The listing builds one solid part. Answer for the finished solid, in the listing's coordinates (mm). Face numbers are marked on the shaded views. A direction names the side the tool comes from. Give positions to 0.01 mm unless a question says otherwise; leave off trailing zeros. Write each loop counter-clockwise with the first axis right and the second up, starting at its lowest first coordinate (ties: lowest second). Pieces come first, ordered by that corner, then holes. Notation, with made-up numbers: (26, -38.5) - (83, -38.5) arc R29 cw to (83, -10.5) - close; hole circle Ø9 at (26, -8.75). An arc over 180 degrees is marked (long way). One line per question, with ' | ' between items. Start each with the question number.
1. A cutting plane is placed at B-B (y = 11.5). Determine the outline of the cut face in (x, z), then the cut area to 3 significant figures.
2. A cutting plane is placed at C-C (z = 5). Determine the outline of the cut face in (x, y), then the cut area to 3 significant figures.
3. A cutting plane is placed at A-A (z = 10.8). Determine the outline of the cut face in (x, y).
4. Find the intervals of material crossed by L1, parallel to X at y = 12, z = 17; L2, parallel to Z at x = -17.5, y = -7.5; L3, parallel to Y at x = -2.2, z = -19.2, in increasing order. Write a range as from..to.
5. Given P1, Ø3.5, axis at x = 21.5, y = 2, coming from the -Z side; P2, Ø7, axis at y = 10.69, z = -19.2, coming from the -X side; P3, Ø11, axis at y = 7.5, z = -20, coming from the +X side, each flat-ended and moving along its own axis, determine where each tip first touches the part or whether it passes through.
6. For the marked faces 1, 2, 3 and 4, determine the directions among +Z, -Z, +X, -X, +Y, -Y from which every point of the face is accessible in a straight line to the end or side of a thin tool.
7. A cutting plane is placed at D-D (x = 11). Determine the outline of the cut face in (y, z), then the cut area to 3 significant figures.
8. The mould has two halves that part along X. Classify the marked faces 5, 6, 7 and 8: +X half, -X half, draft (parallel to the pull), parting line (faces both ways), or undercut.
```python
from build123d import *

# Parameters (mm, degrees)
SKETCH1_R                    = 4
SKETCH1_R_2                  = 2.249999999999999
BOSS_EXTRUDE1_DEPTH          = 24
SKETCH2_R                    = 2.2499999999999956
SKETCH2_R_2                  = 4
BOSS_EXTRUDE2_DEPTH          = 24
CUT_EXTRUDE1_DEPTH           = 14
CUT_EXTRUDE2_START           = -14
CUT_EXTRUDE2_DEPTH           = 14
BOSS_EXTRUDE3_DEPTH          = 2
CUT_EXTRUDE_THIN1_DEPTH      = 70.97528134991671
CUT_EXTRUDE_THIN1_DEPTH_BACK = 53.00000000000001
SKETCH6_W                    = 2
SKETCH6_H                    = 35.40537681916631
SKETCH7_R                    = 2.249999999999999
CUT_EXTRUDE3_DEPTH           = 55.524673314014464
CUT_EXTRUDE4_DEPTH           = 41.99999999999999
CHAMFER2_SIZE                = 1
SKETCH9_R                    = 45.63024731549585
CUT_EXTRUDE5_DEPTH           = 2
SKETCH10_R                   = 89.28313808685371
CUT_EXTRUDE6_DEPTH           = 57.00000000000001
BOSS_EXTRUDE5_START          = 3
SKETCH11_R                   = 3.9999999999999925
BOSS_EXTRUDE5_DEPTH          = 3
BOSS_EXTRUDE6_DEPTH          = 3
BOSS_EXTRUDE7_DEPTH          = 3
CUT_EXTRUDE7_DEPTH           = 56.55663776723714
CUT_EXTRUDE7_DEPTH_BACK      = 56.55663776723714
CUT_EXTRUDE8_START           = -18.000000000000004
CUT_EXTRUDE8_DEPTH           = 18.000000000000004
CHAMFER4_SIZE                = 5


with BuildPart() as part:
    # Sketch1 → Boss-Extrude1 (new body)
    with BuildSketch(Plane.XY):
        with BuildLine():
            Line((0, 15.5), (-30, 15.5))
            Line((-30, 15.5), (-45.50000000000001, 15.499999999999995))
            Line((-45.50000000000001, 15.499999999999995), (-45.5, 1.9e-15))
            ThreePointArc((-45.5, 1.9e-15), (-40.96015510839149, -10.960155108391486), (-30, -15.499999999999996))
            Line((-30, -15.499999999999996), (0, -15.5))
            ThreePointArc((0, -15.5), (10.960155108391488, -10.960155108391486), (15.5, 0))
            Line((15.5, 0), (15.5, 15.5))
            Line((15.5, 15.5), (0, 15.5))
        make_face()
        Circle(SKETCH1_R, mode=Mode.SUBTRACT)
        with Locations((-30, 0)):
            Circle(SKETCH1_R_2, mode=Mode.SUBTRACT)
    extrude(amount=BOSS_EXTRUDE1_DEPTH)

    # Sketch4 → Cut-Extrude2 (cut)
    with BuildSketch(Plane.XY.offset(24).offset(CUT_EXTRUDE2_START)):
        with BuildLine():
            Line((-1.32e-15, 15.499999999999998), (-45.50000000000001, 15.499999999999995))
            Line((-45.50000000000001, 15.499999999999995), (-45.5, 1.9e-15))
            ThreePointArc((-45.5, 1.9e-15), (-40.96015510839149, -10.960155108391486), (-30.000000000000004, -15.5))
            Line((-30.000000000000004, -15.5), (0, -15.5))
            ThreePointArc((0, -15.5), (-15.499999999999998, 1.9e-15), (-1.32e-15, 15.499999999999998))
        make_face()
    extrude(amount=CUT_EXTRUDE2_DEPTH, mode=Mode.SUBTRACT)



with BuildPart() as body_2:
    # Sketch2 → Boss-Extrude2 (new body)
    with BuildSketch(Plane(origin=(0, 0, -2.2), x_dir=(-1, 0, 0), z_dir=(0, 0, -1))):
        with BuildLine():
            Line((-2.85e-15, -15.5), (30.000000000000004, -15.499999999999998))
            ThreePointArc((30.000000000000004, -15.499999999999998), (40.96015510839149, -10.960155108391485), (45.5, 0))
            Line((45.5, 0), (45.50000000000001, 15.499999999999995))
            Line((45.50000000000001, 15.499999999999995), (-15.5, 15.5))
            Line((-15.5, 15.5), (-15.5, 1.73e-15))
            ThreePointArc((-15.5, 1.73e-15), (-10.96015510839149, -10.960155108391486), (-2.85e-15, -15.5))
        make_face()
        with Locations((30, 0)):
            Circle(SKETCH2_R, mode=Mode.SUBTRACT)
        Circle(SKETCH2_R_2, mode=Mode.SUBTRACT)
    extrude(amount=BOSS_EXTRUDE2_DEPTH)

    # Sketch3 → Cut-Extrude1 (cut)
    with BuildSketch(Plane(origin=(0, 0, -26.200000000000003), x_dir=(-1, 0, 0), z_dir=(0, 0, -1))):
        with BuildLine():
            Line((-2.85e-15, -15.5), (30.000000000000004, -15.499999999999998))
            ThreePointArc((30.000000000000004, -15.499999999999998), (40.96015510839149, -10.960155108391485), (45.5, 0))
            Line((45.5, 0), (45.50000000000001, 15.499999999999995))
            Line((45.50000000000001, 15.499999999999995), (1.32e-15, 15.499999999999998))
            ThreePointArc((1.32e-15, 15.499999999999998), (15.5, -3.44e-15), (-2.85e-15, -15.5))
        make_face()
    extrude(amount=-CUT_EXTRUDE1_DEPTH, mode=Mode.SUBTRACT)


with BuildPart() as part_1:
    add(part.part)

    add(body_2.part)  # Boss-Extrude3 merges body 2
    # Sketch5 → Boss-Extrude3 (add)
    with BuildSketch(Plane(origin=(-1.32e-15, 15.499999999999998, 0), x_dir=(1, 1.1e-16, 0), z_dir=(-1.1e-16, 1, 0))):
        Polygon((-45.50000000000001, 12.200000000000001), (1.77e-15, 12.200000000000001), (0, 26.200000000000003), (15.500000000000002, 26.200000000000003), (15.500000000000002, -24), (0, -24), (1.77e-15, -10), (-45.50000000000001, -10), (-45.50000000000001, 0), (-38.50000000000001, 0), (-38.50000000000001, 2.200000000000001), (-45.50000000000001, 2.2), align=None)
    extrude(amount=BOSS_EXTRUDE3_DEPTH)

    # Chamfer1
    # the kernel refuses this chamfer: 10 mm, written as the material it adds along each edge
    with BuildSketch(Plane(origin=(-3.72e-15, 15.5, 10), x_dir=(0.026587242345483465, 0.9996464967899715, 0), z_dir=(0, 0, 1))) as chamfer1_piece_1_section:
        with BuildLine():
            Line((8.29406545002713, 1e-17), (-1.7422154358514688, 6.254838102034438))
            Line((-1.7422154358514688, 6.254838102034438), (-1.9240447967842007, 6.17154294309471))
            ThreePointArc((-1.9240447967842007, 6.17154294309471), (-0.6239231337177482, 3.187248798266774), (-0.19992929935799358, -0.00531744846909673))
            Line((-0.19992929935799358, -0.00531744846909673), (0.00531744846909669, -0.1999292993579943))
            ThreePointArc((0.00531744846909669, -0.1999292993579943), (4.149418712953845, -0.08971011189834381), (8.299382898496228, -0.19992929935799428))
            Line((8.299382898496228, -0.19992929935799428), (8.29406545002713, 1e-17))
        make_face()
    chamfer1_piece_1 = extrude(amount=14, mode=Mode.PRIVATE)
    chamfer1_piece_1 = split(chamfer1_piece_1, bisect_by=Plane(origin=(-2.6872969980278754, 17.5, 17.000000000000004), z_dir=(1.1e-16, -1, 0)), keep=Keep.TOP, mode=Mode.PRIVATE)
    add(chamfer1_piece_1)
    with BuildSketch(Plane(origin=(-1.32e-15, 15.5, -26.200000000000003), x_dir=(-0.9701220678115945, -0.24261733974503139, 0), z_dir=(0, 0, 1))) as chamfer1_piece_2_section:
        with BuildLine():
            Line((6.4929434240243395, 9e-17), (-2.2255005025199233, -7.9899104627409505))
            Line((-2.2255005025199233, -7.9899104627409505), (-2.419524916082242, -7.941386994791944))
            ThreePointArc((-2.419524916082242, -7.941386994791944), (-1.1998107866971348, -3.973182305874418), (-0.19402441356231892, 0.04852346794900628))
            Line((-0.19402441356231892, 0.04852346794900628), (0.0485234679490061, 0.1940244135623182))
            ThreePointArc((0.0485234679490061, 0.1940244135623182), (3.237781752513792, -0.25417376326036684), (6.461492077353489, 0.19751155103585727))
            Line((6.461492077353489, 0.19751155103585727), (6.4929434240243395, 9e-17))
        make_face()
    chamfer1_piece_2 = extrude(amount=14, mode=Mode.PRIVATE)
    chamfer1_piece_2 = split(chamfer1_piece_2, bisect_by=Plane(origin=(-2.687296998027888, 17.5, -19.200000000000006), z_dir=(1.1e-16, -1, 0)), keep=Keep.TOP, mode=Mode.PRIVATE)
    add(chamfer1_piece_2)

    # Sketch6 → Cut-Extrude-Thin1 (cut, two sides: drawn at the far end of the back side and taken through both)
    with BuildSketch(Plane(origin=(0, 0, -26.200000000000003), x_dir=(-1, 0, 0), z_dir=(0, 0, -1)).offset(-CUT_EXTRUDE_THIN1_DEPTH_BACK)):
        with Locations((0, 17.702688409583153)):
            Rectangle(SKETCH6_W, SKETCH6_H)
    extrude(amount=CUT_EXTRUDE_THIN1_DEPTH + CUT_EXTRUDE_THIN1_DEPTH_BACK, mode=Mode.SUBTRACT)

    # Sketch7 → Cut-Extrude3 (cut, symmetric)
    with BuildSketch(Plane(origin=(-1, 0, 0), x_dir=(0, 0, -1), z_dir=(1, 0, 0))):
        with Locations((19.200000000000006, 10.686491673103705)):
            Circle(SKETCH7_R)
    cut_extrude3 = extrude(amount=CUT_EXTRUDE3_DEPTH, both=True, mode=Mode.SUBTRACT)

    # Mirror1: Cut-Extrude3 across plane
    add(cut_extrude3.mirror(Plane(origin=(0, 0, -1.1000000000000003), x_dir=(1, 0, 0), z_dir=(0, 0, -1))), mode=Mode.SUBTRACT)

    # Sketch8 → Cut-Extrude4 (cut)
    with BuildSketch(Plane.ZY.offset(45.50000000000001)):
        Polygon((-15.1788975572378, 12.292958337809747), (-18.58068972058721, 14.97210187210845), (-22.60179216334942, 13.365635207402391), (-23.221102442762213, 9.080025008397632), (-19.8193102794128, 6.4008814740989255), (-15.798207836650597, 8.007348138804984), align=None)
        Polygon((12.978897557237794, 12.292958337809734), (13.598207836650598, 8.007348138804979), (17.61931027941281, 6.400881474098927), (21.02110244276222, 9.080025008397646), (20.401792163349413, 13.365635207402406), (16.38068972058721, 14.972101872108457), align=None)
    extrude(amount=-CUT_EXTRUDE4_DEPTH, mode=Mode.SUBTRACT)

    # Chamfer2
    chamfer2_edges = [part_1.edges().sort_by_distance(p)[0] for p in [
        (-2.449489742783177, -3.1622776601683804, 24),
        (-1.22e-15, -4, -26.2),
    ]]
    chamfer(chamfer2_edges, length=CHAMFER2_SIZE)

    # Sketch9 → Cut-Extrude5 (cut)
    with BuildSketch(Plane(origin=(-1.79e-15, -15.5, 0), x_dir=(-1, 1.2e-16, 0), z_dir=(-1.2e-16, -1, 0))):
        with Locations((14.602356379640469, -2.8500724208981865)):
            Circle(SKETCH9_R)
    extrude(amount=-CUT_EXTRUDE5_DEPTH, mode=Mode.SUBTRACT)

    # Sketch10 → Cut-Extrude6 (cut)
    with BuildSketch(Plane(origin=(0, 0, -12.200000000000001), x_dir=(-1, 0, 0), z_dir=(0, 0, -1))):
        with Locations((18.92287737663878, -1.4489467579892334)):
            Circle(SKETCH10_R)
    extrude(amount=-CUT_EXTRUDE6_DEPTH, mode=Mode.SUBTRACT)

    # Sketch11 → Boss-Extrude5 (add)
    with BuildSketch(Plane.XY.offset(-12.200000000000001).offset(BOSS_EXTRUDE5_START)):
        Polygon((-20.25, 17.499999999999996), (20.250000000000004, 17.499999999999996), (20.250000000000007, -13.499999999999998), (-20.249999999999993, -13.499999999999998), align=None)
        Circle(SKETCH11_R, mode=Mode.SUBTRACT)
    extrude(amount=-BOSS_EXTRUDE5_DEPTH)

    # Sketch13 → Boss-Extrude6 (add)
    with BuildSketch(Plane(origin=(20.250000000000007, 2.27e-15, 0), x_dir=(0, 0, -1), z_dir=(1, 1.1e-16, 0))):
        Polygon((12.200000000000001, 17.499999999999993), (-29.8, 17.499999999999993), (-29.8, -13.500000000000002), (12.200000000000005, -13.500000000000002), align=None)
    extrude(amount=BOSS_EXTRUDE6_DEPTH)

    # Sketch14 → Boss-Extrude7 (add)
    with BuildSketch(Plane.ZY.offset(20.249999999999996)):
        Polygon((-12.200000000000001, -13.499999999999993), (29.8, -13.499999999999993), (29.8, 17.499999999999996), (-12.200000000000001, 17.5), align=None)
    extrude(amount=BOSS_EXTRUDE7_DEPTH)

    # Sketch15 → Cut-Extrude7 (cut, two sides: drawn at the far end of the back side and taken through both)
    with BuildSketch(Plane.ZY.offset(-20.250000000000007).offset(-CUT_EXTRUDE7_DEPTH_BACK)):
        with BuildLine():
            Line((8.05, -0.5000000000000039), (8.05, 4.499999999999997))
            ThreePointArc((8.05, 4.499999999999997), (10.8, 7.249999999999999), (13.550000000000002, 4.499999999999997))
            Line((13.550000000000002, 4.499999999999997), (13.55, -0.5000000000000034))
            ThreePointArc((13.55, -0.5000000000000034), (10.8, -3.2500000000000036), (8.05, -0.5000000000000039))
        make_face()
    extrude(amount=CUT_EXTRUDE7_DEPTH + CUT_EXTRUDE7_DEPTH_BACK, mode=Mode.SUBTRACT)

    # Sketch16 → Cut-Extrude8 (cut)
    with BuildSketch(Plane(origin=(0, 0, -12.200000000000001), x_dir=(-1, 0, 0), z_dir=(0, 0, -1)).offset(CUT_EXTRUDE8_START)):
        with BuildLine():
            Line((-1, 17.499999999999996), (-1, 3.8729833462074166))
            ThreePointArc((-1, 3.8729833462074166), (-4.8e-16, 4), (0.9999999999999991, 3.8729833462074157))
            Line((0.9999999999999991, 3.8729833462074157), (1.0000000000000009, 17.499999999999996))
            Line((1.0000000000000009, 17.499999999999996), (-1, 17.499999999999996))
        make_face()
    extrude(amount=CUT_EXTRUDE8_DEPTH, mode=Mode.SUBTRACT)

    # Chamfer4
    chamfer4_edges = [part_1.edges().sort_by_distance(p)[0] for p in [
        (21.750000000000004, 17.499999999999996, 29.8),
        (21.750000000000007, -13.5, 29.8),
        (-21.749999999999993, -13.499999999999998, 29.8),
        (-21.75, 17.499999999999993, 29.8),
    ]]
    chamfer(chamfer4_edges, length=CHAMFER4_SIZE)


solid = part_1.part
```
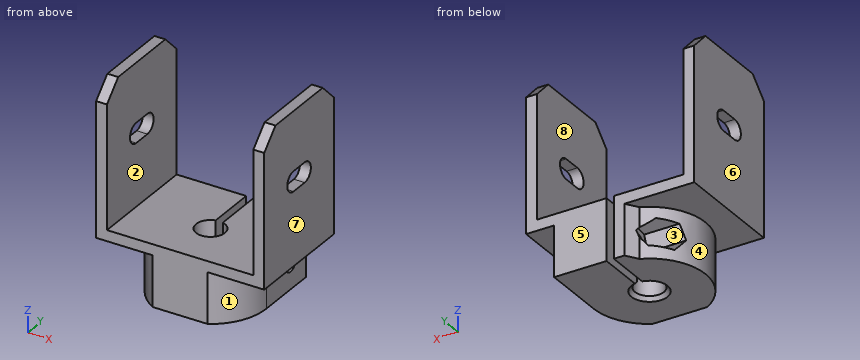
Determined:
1) outline: (-23.25, -12.2) - (-10.39, -12.2) - (-10.39, -15.29) - (-3.5, -15.29) - (-3.5, -17.1) - (-1, -17.1) - (-1, -9.2) - (-20.25, -9.2) - (-20.25, 29.8) - (-23.25, 29.8) - close; (-10.39, -26.2) - (-1, -26.2) - (-1, -21.3) - (-3.5, -21.3) - (-3.5, -22.87) - (-10.39, -22.87) - close; (1, -26.2) - (15.5, -26.2) - (15.5, -21.3) - (1, -21.3) - close; (1, -17.1) - (15.5, -17.1) - (15.5, -12.2) - (23.25, -12.2) - (23.25, 29.8) - (20.25, 29.8) - (20.25, -9.2) - (1, -9.2) - close | area: 578 mm2
2) outline: (-23.25, -13.5) - (-20.25, -13.5) - (-20.25, 17.5) - (-23.25, 17.5) - close; (20.25, -13.5) - (23.25, -13.5) - (23.25, 17.5) - (20.25, 17.5) - close | area: 186 mm2
3) outline: (-23.25, -13.5) - (-20.25, -13.5) - (-20.25, -3.25) - (-23.25, -3.25) - close; (-23.25, 7.25) - (-20.25, 7.25) - (-20.25, 17.5) - (-23.25, 17.5) - close; (20.25, -13.5) - (23.25, -13.5) - (23.25, -3.25) - (20.25, -3.25) - close; (20.25, 7.25) - (23.25, 7.25) - (23.25, 17.5) - (20.25, 17.5) - close
4) L1: -23.25..-20.25, 20.25..23.25 | L2: -12.2..-9.2 | L3: -13.5..-3.34, 3.34..8.44, 12.94..17.5
5) P1: z = -12.2 | P2: x = -3.5 | P3: x = 15.5
6) face 1: -Z, +X, -Y | face 2: +Z, +Y, -Y | face 3: -X | face 4: -Z, -X
7) outline: (-13.5, -12.2) - (-10.92, -12.2) - (-10.92, -26.2) - (17.5, -26.2) - (17.5, -9.2) - (-13.5, -9.2) - close; hole circle Ø4.5 at (10.69, -19.2) | area: 475 mm2
8) face 5: draft | face 6: -X half | face 7: +X half | face 8: undercut
